Geometry check sheet. Reference: drawing and pictorial views, mm from the part's lowest x, y, z. A direction names the side the tool comes from. Round coordinates to 2 decimals unless told otherwise and drop trailing zeros. Write each loop counter-clockwise with the first axis right and the second up, starting at its lowest first coordinate (ties: lowest second). Pieces come first, ordered by that corner, then holes. Notation, with made-up numbers: M -29.5,87 L -11.5,87 A26 cw -11.5,117 Z; hole C 73,83.25 d8. An arc over 180 degrees is marked long. Answer in a Markdown table with one row per item.
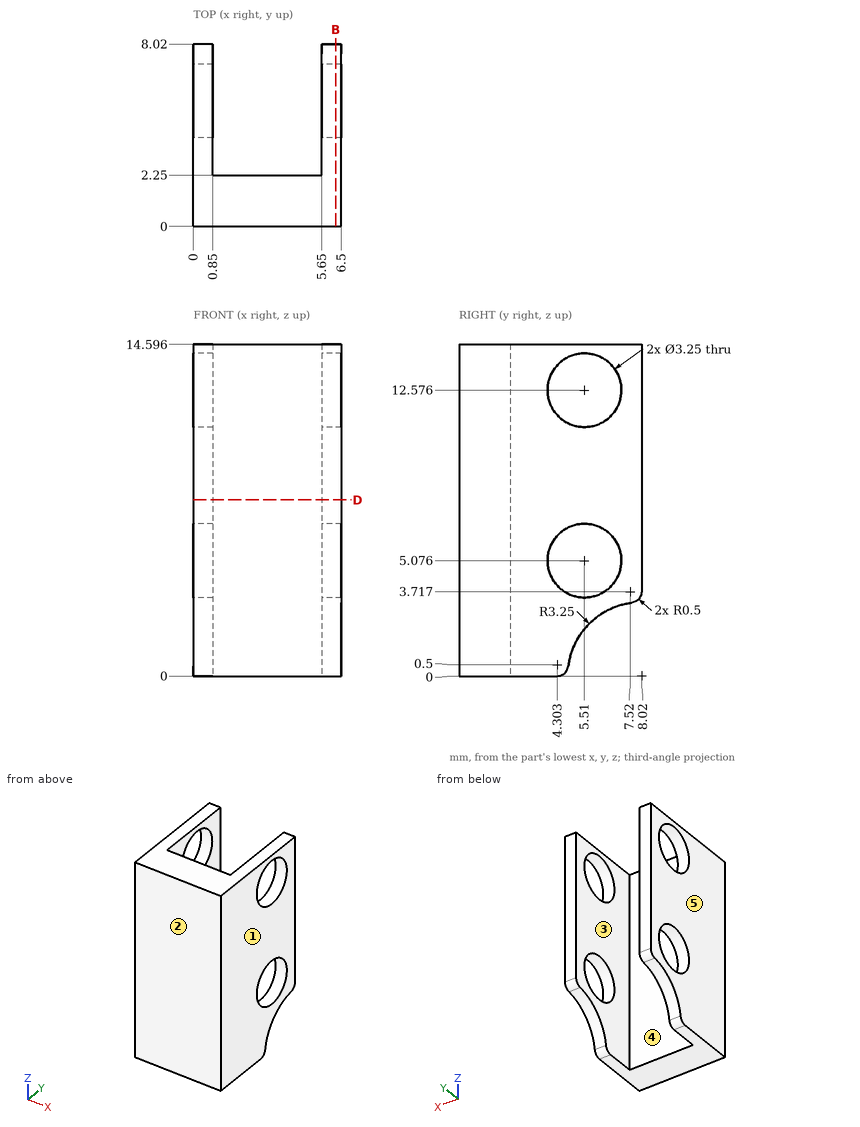
1. Section check B-B, the plane x = 6.25. Count the separate pieces of the cut face and the enclosed holes in it.
Found:
| item | result |
|---|---|
| separate pieces | 1 |
| enclosed holes | 2 |
2. Scan lines: L1, parallel to X at y = 3.25, z = 9.75; L2, parallel to Z at x = 6.25, y = 6 (1 decimal); L3, parallel to Y at x = 1, z = 1.5. Record each from-to range of solid material in increasing order.
Found:
| item | result |
|---|---|
| L1 | x = 0 to 0.85, 5.65 to 6.5 |
| L2 | z = 2.5 to 3.5, 6.6 to 11, 14.1 to 14.6 |
| L3 | y = 0 to 2.25 |
3. Draft check along X on the marked faces 1, 2 and 3. Enter one of: +X half, -X half, draft (parallel to the pull), parting line (faces both ways), or undercut.
Found:
| item | result |
|---|---|
| face 1 | +X half |
| face 2 | draft |
| face 3 | undercut |
4. Access from +Z, -Z, +X, -X, +Y, -Y to the whole of each face (thin tool, end or side, straight path). Record for the marked faces 4 and 5.
Found:
| item | result |
|---|---|
| face 4 | +Z, -Z, +Y |
| face 5 | +Z, -Z, -X, +Y, -Y |
5. Section check D-D, the plane z = 7.75. Record the cut outline in (x, y).
Found:
| item | result |
|---|---|
| outline | M 0,0 L 6.5,0 L 6.5,8.02 L 5.65,8.02 L 5.65,2.25 L 0.85,2.25 L 0.85,8.02 L 0,8.02 Z |
6. Go/stop test with flat-tipped pins: pin 1 (3.5 mm diameter, centred on y = 5.51, z = 5.08, fed in from -X); pin 2 (1.4 mm diameter, centred on x = 3, z = 4, fed in from +Y). Record where each tip stops, or that it passes through.
Found:
| item | result |
|---|---|
| pin 1 | stops at x = 0 |
| pin 2 | stops at y = 2.25 |
